Part model, mm, in its own coordinate system. Round coordinates to 2 decimals unless told otherwise and drop trailing zeros. Write each loop counter-clockwise with the first axis right and the second up, starting at its lowest first coordinate (ties: lowest second). Pieces come first, ordered by that corner, then holes. Notation, with made-up numbers: M -23,18 L 17,18 A27 ccw 17,50 Z; hole C 59.25,13 d5. An arc over 180 degrees is marked long. Use one line per item in the form item = value. Start each with the question number.
Item 1: Cut at A-A, the plane z = 0.6. Give the cut face in (x, y), then the cut area to 3 significant figures.
Item 2: Probe L1, parallel to Y at x = -27, z = 0.5; L2, parallel to X at y = -197.5, z = 1.25; L3, parallel to X at y = 137.5, z = 1.05. List the from-to ranges inside material, lowest first.
Item 3: Flat gauge pin, fed straight in: pin 1 Ø1 at (x, z) = (-145, 1) entering from +Y. Where does the tip first touch, or does it go through?
Autodesk Inventor part; units mm, degrees
ref_plane "YZ Plane" through (0, 0, 0) normal (1, 0, 0) x (0, 1, 0)
ref_plane "XZ Plane" through (0, 0, 0) normal (0, 1, 0) x (-1, 0, 0)
ref_plane "XY Plane" through (0, 0, 0) normal (0, 0, 1) x (1, 0, 0)
sketch "Esquisse1" plane through (0, 0, 0) normal (0, 0, 1) x (1, 0, 0)
  line L0 (-366.5, -212.5) -> (368.5, -212.5)
  line L1 (368.5, -212.5) -> (368.5, 152.5)
  line L2 (368.5, 152.5) -> (-366.5, 152.5)
  line L3 (-366.5, 152.5) -> (-366.5, -212.5)
  line L4 (-366.5, -212.5) -> (368.5, 152.5) construction
  line L5 (-354, -200) -> (356, -200)
  line L6 (356, -200) -> (356, 140)
  line L7 (356, 140) -> (-354, 140)
  line L8 (-354, 140) -> (-354, -200)
  line L9 (-354, -200) -> (356, 140) construction
  circle A0 centre (-351.5, 137.5) radius 2.5
  circle A1 centre (-351.5, -197.5) radius 2.5
  circle A2 centre (353.5, -197.5) radius 2.5
  circle A3 centre (353.5, 137.5) radius 2.5
  point P0 (-354, -197.5)
  point P1 (-351.5, -200)
  point P2 (353.5, -200)
  point P3 (356, -197.5)
  point P4 (356, 137.5)
  point P5 (353.5, 140)
  point P6 (-354, 137.5)
  point P7 (-351.5, 140)
  dimension "d0" = 735
  dimension "d1" = 365
  dimension "d2" = 12.5
  dimension "d3" = 12.5
  dimension "d4" = 5
  dimension "d7" = 5
  dimension "d8" = 5
  dimension "d9" = 5
  dimension "d75" = 12.5
  dimension "d76" = 12.5
extrude "Extrusion1" add sketch "Esquisse1" along normal blind 2 contours L3 L2 L1 L0 | L8 A1 L5 | A1 L8 A0 L7 A3 L6 A2 L5 | A2 L6 L5 | L8 L7 A0 | A3 L7 L6
sketch "Esquisse3" plane through (0, 0, 2) normal (0, 0, 1) x (1, 0, 0)
  line L0 (-194, 155.1637) -> (-44, 155.1637)
  line L1 (-44, 155.1637) -> (-44, 102.5)
  line L2 (-44, 102.5) -> (-194, 102.5)
  line L3 (-194, 102.5) -> (-194, 155.1637)
  line L4 (368.5, -212.5) -> (368.5, 152.5)
  line L5 (368.5, 152.5) -> (-366.5, 152.5)
  point P0 (0, 0)
  point P1 (-44, 128.8319)
  dimension "d65" = 412.5
  dimension "d66" = 150
  dimension "d67" = 50
extrude "Extrusion2" cut sketch "Esquisse3" against normal through all
sketch "Esquisse4" plane through (0, 0, 2) normal (0, 0, 1) x (1, 0, 0)
  circle A0 centre (-27, 137.5) radius 2.5
  circle A1 centre (-27, -197.5) radius 2.5
  line L0 (-29.5, 269.4833) -> (-29.5, -384.936)
  line L1 (368.5, -212.5) -> (368.5, 152.5)
  circle A2 centre (-351.5, -197.5) radius 2.5
  circle A3 centre (-351.5, 137.5) radius 2.5
  point P0 (0, 0)
  dimension "d68" = 5
  dimension "d69" = 5
  dimension "d70" = 398
  dimension "d71" = 0
  dimension "d72" = 0
extrude "Extrusion3" cut sketch "Esquisse4" along normal through all both and the other way through all contours A0 | A1
properties part number "PlaqueLargeur"
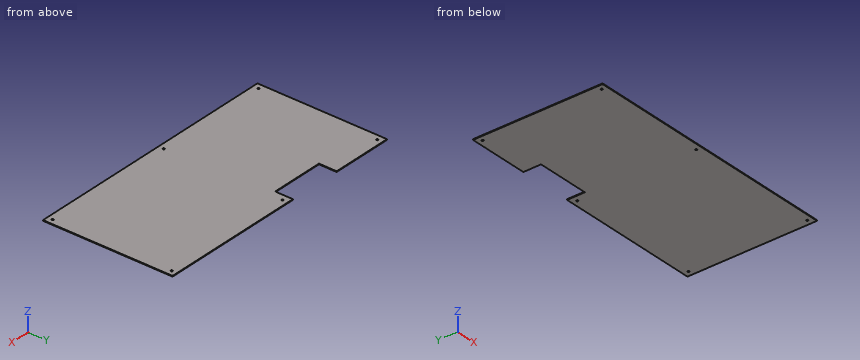
Model answer:
q1.outline = M -366.5,-212.5 L 368.5,-212.5 L 368.5,152.5 L -44,152.5 L -44,102.5 L -194,102.5 L -194,152.5 L -366.5,152.5 Z; hole C -351.5,-197.5 d5; hole C -351.5,137.5 d5; hole C -27,-197.5 d5; hole C -27,137.5 d5; hole C 353.5,-197.5 d5; hole C 353.5,137.5 d5
q1.area = 261,000 mm²
q2.L1 = -212.5 to -200, -195 to 135, 140 to 152.5
q2.L2 = -366.5 to -354, -349 to -29.5, -24.5 to 351, 356 to 368.5
q2.L3 = -366.5 to -354, -349 to -194, -44 to -29.5, -24.5 to 351, 356 to 368.5
q3.pin_1 = 102.5
